Model file for the job. Use its own axes, mm. Face numbers are marked on the shaded views. Coordinates: 2 decimals unless noted, no trailing zeros. Write each loop counter-clockwise with the first axis right and the second up, starting at its lowest first coordinate (ties: lowest second). Pieces come first, ordered by that corner, then holes. Notation, with made-up numbers: (57.25, 61) -> (67.25, 61) arc R9 ccw to (67.25, 73) -> close; hole circle Ø4 at (73.5, 54). An arc over 180 degrees is marked (long way). Write item = value, one per line. Start each with the question number.
from build123d import *

# Parameters (mm, degrees)
SKETCH1_R           = 21.25
SKETCH1_R_2         = 2.5
BOSS_EXTRUDE1_DEPTH = 74
FILLET1_R           = 6
SKETCH2_R           = 17.145
SKETCH2_R_2         = 4.445
CUT_EXTRUDE1_DEPTH  = 65


with BuildPart() as part:
    # Sketch1 → Boss-Extrude1 (new body)
    with BuildSketch(Plane.XY):
        Circle(SKETCH1_R)
        Circle(SKETCH1_R_2, mode=Mode.SUBTRACT)
    extrude(amount=BOSS_EXTRUDE1_DEPTH)

    # Fillet1
    fillet1_edges = [part.edges().sort_by_distance(p)[0] for p in [
        (-21.25, 0, 74),
    ]]
    fillet(fillet1_edges, radius=FILLET1_R)

    # Sketch2 → Cut-Extrude1 (cut)
    with BuildSketch(Plane(origin=(0, 0, 0), x_dir=(-1, 0, 0), z_dir=(0, 0, -1))):
        Circle(SKETCH2_R)
        Circle(SKETCH2_R_2, mode=Mode.SUBTRACT)
    extrude(amount=-CUT_EXTRUDE1_DEPTH, mode=Mode.SUBTRACT)


solid = part.part
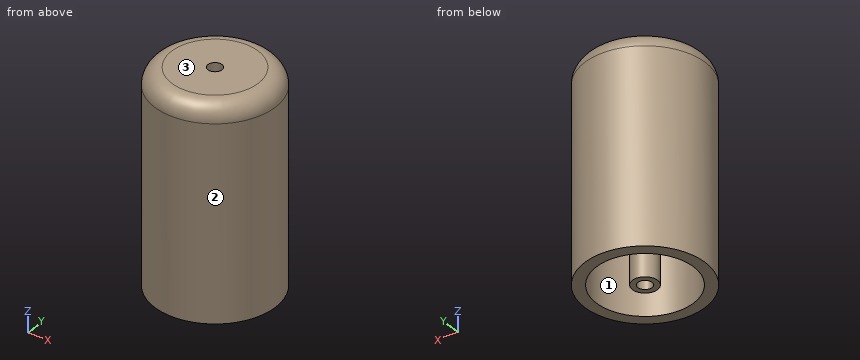
(1) Drop flat-ended pins along their axis: pin 1 Ø2 at (y, z) = (7.5, 21.5) entering from -X; pin 2 Ø6 at (x, z) = (11.5, 64.5) entering from +Y; pin 3 Ø1 at (x, z) = (2, 12.5) entering from -Y. Give the stop position or say it passes through.
(2) Mould opens along Y. For the marked faces 1, 2 and 3 say: released by +Y, released by -Y, zero draft, split by the parting line, or undercut.
(3) Drill centre lines: line 1 along Y through (x, z) = (0, 38) (3 decimals); line 2 along X through (y, z) = (-4, 48); line 3 along Y through (x, z) = (0.5, 32). Where is each one in solid material? Low to high.
(4) Saw through at A-A (y = 0). Give the cut face in (x, z) (3 decimals).
(5) Saw through at C-C (z = 5.5). Give the cut face in (x, y) (3 decimals), then the cut area to 3 significant figures.
Returned:
q1.pin_1 = -20.23
q1.pin_2 = 19.48
q1.pin_3 = -21.2
q2.face_1 = undercut
q2.face_2 = split by the parting line
q2.face_3 = zero draft
q3.line_1 = -21.25 to -17.145, -4.445 to -2.5, 2.5 to 4.445, 17.145 to 21.25
q3.line_2 = -20.87 to -16.67, -1.94 to 1.94, 16.67 to 20.87
q3.line_3 = -21.24 to -17.14, -4.42 to -2.45, 2.45 to 4.42, 17.14 to 21.24
q4.outline = (-21.25, 0) -> (-17.145, 0) -> (-17.145, 65) -> (-4.445, 65) -> (-4.445, 0) -> (-2.5, 0) -> (-2.5, 74) -> (-15.25, 74) arc R6 ccw to (-21.25, 68) -> close; (2.5, 0) -> (4.445, 0) -> (4.445, 65) -> (17.145, 65) -> (17.145, 0) -> (21.25, 0) -> (21.25, 68) arc R6 ccw to (15.25, 74) -> (2.5, 74) -> close
q5.outline = circle Ø42.5 at (0, 0); circle Ø8.89 at (0, 0); hole circle Ø34.29 at (0, 0); hole circle Ø5 at (0, 0)
q5.area = 538 mm2
